Autodesk Fusion 360 part; units mm, degrees
sketch "Sketch1" plane through (0, 0, 0) normal (0, 0, 1) x (1, 0, 0)
  line L0 (10, -10) -> (-10, -10)
  line L1 (-10, -10) -> (-10, 10)
  line L2 (-10, 10) -> (10, 10)
  line L3 (10, 10) -> (10, -10)
  line L4 (10, -10) -> (-10, 10) construction
  line L5 (-10, -10) -> (10, 10) construction
  line L6 (10.3, -10.3) -> (-10.3, -10.3)
  line L7 (-10.3, -10.3) -> (-10.3, 10.3)
  line L8 (-10.3, 10.3) -> (10.3, 10.3)
  line L9 (10.3, 10.3) -> (10.3, -10.3)
  line L10 (-14.3, -14.3) -> (-14.3, 14.3)
  line L11 (-14.3, 14.3) -> (14.3, 14.3)
  line L12 (14.3, 14.3) -> (14.3, -14.3)
  line L13 (14.3, -14.3) -> (-14.3, -14.3)
  line L14 (-14.3, -14.3) -> (14.3, -14.3)
  line L15 (14.3, -14.3) -> (14.3, -18.3)
  line L16 (14.3, -18.3) -> (-14.3, -18.3)
  line L17 (-14.3, -18.3) -> (-14.3, -14.3)
  dimension "d1" = 20
  dimension "d2" = 20
  dimension "d3" = -0.3
  dimension "d4" = -4.3
  dimension "d10" = 28.6
  dimension "d11" = 4
extrude "Extrude1" add sketch "Sketch1" along normal blind 25 contours L10 L11 L12 L13 L14 | L13 L14 L15 L16 L17
sketch "Sketch3" plane through (0, -10.3, 0) normal (0, 1, 0) x (-1, 0, 0)
  line L0 (-10.3, 0) -> (10.3, 0)
  line L1 (10.3, 0) -> (10.3, 25)
  line L2 (10.3, 25) -> (-10.3, 25)
  line L3 (-10.3, 25) -> (-10.3, 0)
  line L4 (-10.3, 25) -> (10.3, 25)
  line L5 (10.3, 25) -> (10.3, 0)
  line L6 (10.3, 0) -> (-10.3, 0)
  line L7 (-10.3, 0) -> (-10.3, 25)
  line L8 (-10.3, 25) -> (10.3, 0) construction
  line L9 (10.3, 25) -> (-10.3, 0) construction
  line L10 (2.1073, 8.85) -> (4.2147, 12.5)
  line L11 (4.2147, 12.5) -> (2.1073, 16.15)
  line L12 (2.1073, 16.15) -> (-2.1073, 16.15)
  line L13 (-2.1073, 16.15) -> (-4.2147, 12.5)
  line L14 (-4.2147, 12.5) -> (-2.1073, 8.85)
  line L15 (-2.1073, 8.85) -> (2.1073, 8.85)
  circle A0 centre (0, 12.5) radius 2.1
  point P0 (0, 12.5)
  dimension "d12" = 25
  dimension "d13" = 3.65
  dimension "d16" = 4.2
extrude "Extrude4" cut sketch "Sketch3" against normal blind 8 contours A0
extrude "Extrude3" cut sketch "Sketch3" against normal blind 4 contours L10 L11 L12 L13 L14 L15 | A0
sketch "Sketch6" plane through (0, 14.3, 0) normal (0, 1, 0) x (-1, 0, 0)
  line L0 (-14.3, 0) -> (14.3, 0)
  line L1 (14.3, 0) -> (14.3, 25)
  line L2 (14.3, 25) -> (-14.3, 25)
  line L3 (-14.3, 25) -> (-14.3, 0)
  line L4 (-14.3, 25) -> (14.3, 0) construction
  line L5 (14.3, 25) -> (-14.3, 0) construction
  line L6 (7.5, 25) -> (-7.5, 25)
  line L7 (-7.5, 25) -> (-7.5, 0)
  line L8 (-7.5, 0) -> (7.5, 0)
  line L9 (7.5, 0) -> (7.5, 25)
  line L10 (7.5, 25) -> (-7.5, 0) construction
  line L11 (-7.5, 25) -> (7.5, 0) construction
  point P0 (0, 12.5)
  dimension "d35" = 15
  dimension "d36" = 25
extrude "Extrude10" add sketch "Sketch6" along normal blind 30 contours L0 L2 L6 L7 L8 L9
sketch "Sketch7" plane through (-7.5, 0, 0) normal (-1, 0, 0) x (0, -1, 0)
  line L0 (-14.3, 0) -> (-14.3, 25)
  line L1 (-14.3, 25) -> (-44.3, 25)
  line L2 (-44.3, 25) -> (-44.3, 0)
  line L3 (-44.3, 0) -> (-14.3, 0)
  line L4 (-14.3, 25) -> (-44.3, 0) construction
  line L5 (-44.3, 25) -> (-14.3, 0) construction
  circle A0 centre (-29.3, 12.5) radius 2.1
  line L6 (-27.1927, 8.85) -> (-25.0853, 12.5)
  line L7 (-25.0853, 12.5) -> (-27.1927, 16.15)
  line L8 (-27.1927, 16.15) -> (-31.4073, 16.15)
  line L9 (-31.4073, 16.15) -> (-33.5147, 12.5)
  line L10 (-33.5147, 12.5) -> (-31.4073, 8.85)
  line L11 (-31.4073, 8.85) -> (-27.1927, 8.85)
  line L12 (-29.3, 5.75) -> (-23.4543, 9.125)
  line L13 (-23.4543, 9.125) -> (-23.4543, 15.875)
  line L14 (-23.4543, 15.875) -> (-29.3, 19.25)
  line L15 (-29.3, 19.25) -> (-35.1457, 15.875)
  line L16 (-35.1457, 15.875) -> (-35.1457, 9.125)
  line L17 (-35.1457, 9.125) -> (-29.3, 5.75)
  line L18 (-24.4543, 15.2976) -> (-29.3, 18.0953)
  line L19 (-29.3, 18.0953) -> (-34.1457, 15.2976)
  line L20 (-34.1457, 15.2976) -> (-34.1457, 9.7024)
  line L21 (-34.1457, 9.7024) -> (-29.3, 6.9047)
  line L22 (-29.3, 6.9047) -> (-24.4543, 9.7024)
  line L23 (-24.4543, 9.7024) -> (-24.4543, 15.2976)
  point P0 (-29.3, 12.5)
  point P1 (-29.3, 12.5)
  point P2 (-29.3, 12.5)
  dimension "d43" = 4.2
  dimension "d50" = 3.65
  dimension "d54" = 6.75
  dimension "d55" = -1
extrude "Extrude13" cut sketch "Sketch7" along normal blind 4 from surface at -15 contours L6 L7 L8 L9 L10 L11
extrude "Extrude12" cut sketch "Sketch7" against normal blind 15 contours A0
extrude "Extrude11" add sketch "Sketch7" along normal blind 1.5 contours L12 L13 L14 L15 L16 L17
fillet "Fillet1" radius 3.5 2 edges at (-7.5, 44.3, 12.5) (7.5, 44.3, 12.5)
fillet "Fillet2" radius 2 2 edges at (-7.5, 14.3, 12.5) (7.5, 14.3, 12.5)
fillet "Fillet3" radius 2 4 edges at (-14.3, 14.3, 12.5) (-14.3, -18.3, 12.5) (14.3, -18.3, 12.5) (14.3, 14.3, 12.5)
chamfer "Chamfer1" distance 1 angle 45 32 edges at (-13.7142, -17.7142, 25) (0, -18.3, 25) (13.7142, -17.7142, 25) (14.3, -2, 25) (13.7142, 13.7142, 25) (10.9, 14.3, 25) (8.0858, 14.8858, 25) (7.5, 28.55, 25) (6.4749, 43.2749, 25) (0, 44.3, 25) (-6.4749, 43.2749, 25) (-7.5, 28.55, 25) (-8.0858, 14.8858, 25) (-10.9, 14.3, 25) (-13.7142, 13.7142, 25) (-14.3, -2, 25) (-13.7142, 13.7142, 0) (-10.9, 14.3, 0) (-8.0858, 14.8858, 0) (-7.5, 28.55, 0) (-6.4749, 43.2749, 0) (0, 44.3, 0) (6.4749, 43.2749, 0) (7.5, 28.55, 0) (8.0858, 14.8858, 0) (10.9, 14.3, 0) (13.7142, 13.7142, 0) (14.3, -2, 0) (13.7142, -17.7142, 0) (0, -18.3, 0) (-13.7142, -17.7142, 0) (-14.3, -2, 0)
equation "d35 = 28.6 mm - 4 mm - 4 mm - 0.6 mm - 5 mm"
equation "d54 = ( 13.5 / 2 ) * 1 mm"
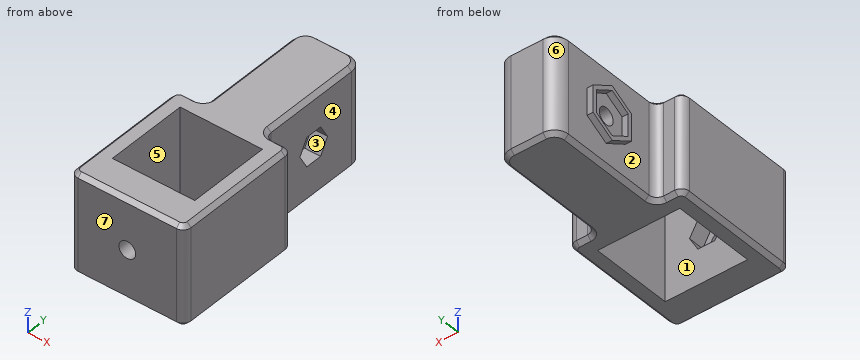
CAD build for the part. Positions are in the model's coordinates, mm. Face numbers are marked on the shaded views. A direction names the side the tool comes from. Coordinates: 2 decimals unless noted, no trailing zeros. Order: outer loops, then holes, each group sorted by start corner. A loop starts at its lowest first (then second) coordinate and runs counter-clockwise, first axis right, second up. Notation, with made-up numbers: (86, -28.75) - (92, -28.75) arc R5 ccw to (92, -21.75) - close; hole circle Ø4 at (32.25, -6). An arc over 180 degrees is marked (long way). Use a Markdown table: item, result. Add a question column.
(1) Saw through at C-C (z = 8). Give the cut face in (x, y).
(2) Drill centre lines: line 1 along Z through (x, y) = (0, -16.5); line 2 along X through (y, z) = (7.5, 9.25); line 3 along Y through (x, z) = (0, 2.5). Where is each one in solid material? Low to high. Write a range as [from, to].
(3) Flat gauge pins, fed straight in: pin 1 (6 mm diameter, centred on y = 21, z = 12.5, fed in from -X); pin 2 (11.5 mm diameter, centred on y = 32, z = 13.5, fed in from +X); pin 3 (6 mm diameter, centred on x = 3, y = -4.5, fed in from +Z); pin 4 (3 mm diameter, centred on y = 31.5, z = 14, fed in from -X). Where does each tip first touch, or does it go through?
(4) Pull direction Y, two halves, no side cores. Call the marked faces 5, 6 and 7: +Y half, -Y half, draft (parallel to the pull), parting line (faces both ways), or undercut.
(5) Saw through at A-A (x = 0). Give the cut face in (y, z).
(6) Which spindle directions (+Z, -Z, +X, -X, +Y, -Y) get a long thin tool onto all of the face, cutting with end or side? Do the marked faces 1, 2, 3 and 4. Say none if no direction does.
(7) Saw through at D-D (x = 11). Give the cut face in (y, z).
(8) Saw through at B-B (y = 18). Give the cut face in (x, z), then the cut area to 3 significant figures.
Solved:
| question | item | result |
|---|---|---|
| 1 | outline | (-14.3, -16.3) arc R2 ccw to (-12.3, -18.3) - (12.3, -18.3) arc R2 ccw to (14.3, -16.3) - (14.3, 12.3) arc R2 ccw to (12.3, 14.3) - (9.5, 14.3) arc R2 cw to (7.5, 16.3) - (7.5, 40.8) arc R3.5 ccw to (4, 44.3) - (-4, 44.3) arc R3.5 ccw to (-7.5, 40.8) - (-7.5, 33.2) - (-9, 33.2) - (-9, 31.2) - (-7.5, 31.2) - (-7.5, 27.4) - (-9, 27.4) - (-9, 25.4) - (-7.5, 25.4) - (-7.5, 16.3) arc R2 cw to (-9.5, 14.3) - (-12.3, 14.3) arc R2 ccw to (-14.3, 12.3) - close; hole (-10.3, -10.3) - (10.3, -10.3) - (10.3, 10.3) - (-10.3, 10.3) - close |
| 2 | line 1 | z = [0, 10.4], [14.6, 25] |
| 2 | line 2 | x = [-14.3, -10.3], [10.3, 14.3] |
| 2 | line 3 | y = [-18.3, -10.3], [10.3, 44.3] |
| 3 | pin 1 | stops at x = -9 |
| 3 | pin 2 | stops at x = 7.5 |
| 3 | pin 3 | passes through |
| 3 | pin 4 | stops at x = -7.5 |
| 4 | face 5 | undercut |
| 4 | face 6 | +Y half |
| 4 | face 7 | -Y half |
| 5 | outline | (-18.3, 1) - (-17.3, 0) - (-10.3, 0) - (-10.3, 8.85) - (-14.3, 8.85) - (-14.3, 10.4) - (-18.3, 10.4) - close; (-18.3, 14.6) - (-14.3, 14.6) - (-14.3, 16.15) - (-10.3, 16.15) - (-10.3, 25) - (-17.3, 25) - (-18.3, 24) - close; (10.3, 0) - (43.3, 0) - (44.3, 1) - (44.3, 24) - (43.3, 25) - (10.3, 25) - close; hole circle Ø4.2 at (29.3, 12.5) |
| 6 | face 1 | +Z, -Z |
| 6 | face 2 | -X |
| 6 | face 3 | +X |
| 6 | face 4 | +Z, -Z, +X, +Y |
| 7 | outline | (-18.3, 1) - (-17.3, 0) - (13.3, 0) - (14.3, 1) - (14.3, 24) - (13.3, 25) - (-17.3, 25) - (-18.3, 24) - close |
| 8 | outline | (-7.5, 1) - (-6.5, 0) - (6.5, 0) - (7.5, 1) - (7.5, 24) - (6.5, 25) - (-6.5, 25) - (-7.5, 24) - close |
| 8 | area | 373 mm² |
